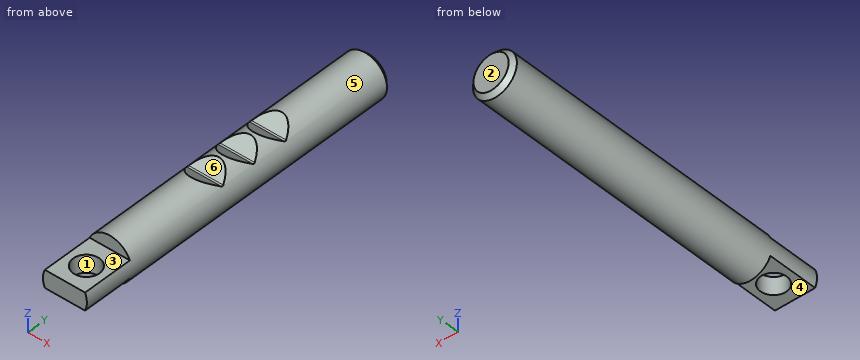
```python
from build123d import *

# Parameters (mm, degrees)
F0_R          = 10
F1_DEPTH      = 156
F2_SIZE       = 2
F3_W          = 20
F3_H          = 8
F4_DEPTH      = 23
F5_R          = 6
F6_DEPTH      = 10.001
F6_DEPTH_BACK = 10.001
F8_DEPTH      = 10.001
F8_DEPTH_BACK = 10.001


# Not quite as in the source:
# - a pattern or mirror of a feature is missing from the dataset's text; its kind, count and spacing are read off the source's solid


with BuildPart() as f1:
    # F0 (on Front) → F1 (new body)
    with BuildSketch(Plane.XZ):
        Circle(F0_R)
    extrude(amount=-F1_DEPTH)

    # F2
    f2_edges = [f1.edges().sort_by_distance(p)[0] for p in [
        (-10, 156, 0),
    ]]
    chamfer(f2_edges, length=F2_SIZE)

    # F3 (on Front) → F4 (cut)
    with BuildSketch(Plane.XZ):
        with Locations((0, 8)):
            Rectangle(F3_W, F3_H)
    f4 = extrude(amount=-F4_DEPTH, mode=Mode.SUBTRACT)

    # F4_copies: F4 across plane
    add(f4.mirror(Plane(origin=(0, 0, 0), x_dir=(-1, 0, 0), z_dir=(0, 0, -1))), mode=Mode.SUBTRACT)

    # F5 (on Top) → F6 (cut, two sides)
    with BuildSketch(Plane.XY) as f6_sk:
        with Locations((0, 11)):
            Circle(F5_R)
    extrude(amount=-F6_DEPTH, mode=Mode.SUBTRACT)
    extrude(f6_sk.sketch, amount=F6_DEPTH_BACK, mode=Mode.SUBTRACT)

    # F7 (on Right) → F8 (cut, two sides)
    with BuildSketch(Plane.YZ) as f8_sk:
        with BuildLine():
            Line((96.0621778265, 10.5), (79.9378221735, 10.5))
            Line((79.9378221735, 10.5), (87.5, 6.1339745962))
            ThreePointArc((87.5, 6.1339745962), (88, 6), (88.5, 6.1339745962))
            Line((88.5, 6.1339745962), (96.0621778265, 10.5))
        make_face()
        with BuildLine():
            Line((112.1865334795, 10.5), (96.0621778265, 10.5))
            Line((96.0621778265, 10.5), (103.624355653, 6.1339745962))
            ThreePointArc((103.624355653, 6.1339745962), (104.124355653, 6), (104.624355653, 6.1339745962))
            Line((104.624355653, 6.1339745962), (112.1865334795, 10.5))
        make_face()
        with BuildLine():
            Line((72.375644347, 6.1339745962), (79.9378221735, 10.5))
            Line((79.9378221735, 10.5), (63.8134665205, 10.5))
            Line((63.8134665205, 10.5), (71.375644347, 6.1339745962))
            ThreePointArc((71.375644347, 6.1339745962), (71.875644347, 6), (72.375644347, 6.1339745962))
        make_face()
    extrude(amount=-F8_DEPTH, mode=Mode.SUBTRACT)
    extrude(f8_sk.sketch, amount=F8_DEPTH_BACK, mode=Mode.SUBTRACT)


solid = f1.part
```
The listing builds one solid part. Answer for the finished solid, in the listing's coordinates (mm). Face numbers are marked on the shaded views. A direction names the side the tool comes from. Round coordinates to 2 decimals unless told otherwise and drop trailing zeros. Loops run counter-clockwise (first coordinate to the right, second up) from the corner with the lowest first, then second, coordinate; pieces in that order, holes last. Notation, with made-up numbers: (27.5, 32.5) - (38.5, 32.5) arc R28 ccw to (38.5, 68.5) - close; hole circle Ø7 at (68.5, 6). An arc over 180 degrees is marked (long way). Return JSON: item names as keys, results as strings. Group by question number.
1. The part is cut by section D-D on y = 131.5. Determine the outline of the cut face in (x, z), then the cut area to 3 significant figures.
2. Each of these flat-tipped pins is pushed along its axis until it touches: P1, Ø12, axis at x = -3.5, z = 1.5, coming from the -Y side; P2, Ø1.5, axis at x = 4.5, z = 5.5, coming from the -Y side; P3, Ø1.5, axis at y = 138.5, z = 4, coming from the -X side; P4, Ø10, axis at x = -7.5, y = 84.5, coming from the +Z side. Where does it stop, or does it pass through?
3. The part is cut by section C-C on z = 0. Determine the outline of the cut face in (x, y), then the cut area to 3 significant figures.
4. Consider probe 1 along X at (y, z) = (11, 0.5); probe 2 along Y at (x, z) = (0, 1.5); probe 3 along Y at (x, z) = (-4, 7.75). Determine where each line is inside the solid, lowest interval first.
5. The part is cut by section B-B on x = 0. Determine the outline of the cut face in (y, z), then the cut area to 3 significant figures.
6. The mould has two halves that part along Y. Classify the marked faces 1, 2 and 3: pulls with the +Y half, pulls with the -Y half, needs draft (parallel to the pull), parting line crosses it, or undercut.
7. The part is cut by section A-A on y = 11. Determine the outline of the cut face in (x, z).
8. Which of the six approach directions +Z, -Z, +X, -X, +Y, -Y give full straight-line access (tool end or side, diameter ignored) to the marked faces 4, 5 and 6?
Resolved:
{
 "1": {"outline": "circle Ø20 at (0, 0)", "area": "314 mm²"},
 "2": {"P1": "stops at y = 0", "P2": "stops at y = 23", "P3": "stops at x = -9.46", "P4": "stops at z = 9.44"},
 "3": {"outline": "(-10, 0) - (10, 0) - (10, 154) - (8, 156) - (-8, 156) - (-10, 154) - close; hole circle Ø12 at (0, 11)", "area": "3,000 mm²"},
 "4": {"probe 1": "x = -9.99 to -6, 6 to 9.99", "probe 2": "y = 0 to 5, 17 to 156", "probe 3": "y = 23 to 68.58, 75.17 to 84.7, 91.3 to 100.83, 107.42 to 155.28"},
 "5": {"outline": "(0, -4) - (5, -4) - (5, 4) - (0, 4) - close; (17, -4) - (23, -4) - (23, -10) - (154, -10) - (156, -8) - (156, 8) - (154, 10) - (111.32, 10) - (104.62, 6.13) arc R1 cw to (103.62, 6.13) - (96.93, 10) - (95.2, 10) - (88.5, 6.13) arc R1 cw to (87.5, 6.13) - (80.8, 10) - (79.07, 10) - (72.38, 6.13) arc R1 cw to (71.38, 6.13) - (64.68, 10) - (23, 10) - (23, 4) - (17, 4) - close", "area": "2,650 mm²"},
 "6": {"face 1": "undercut", "face 2": "pulls with the +Y half", "face 3": "needs draft"},
 "7": {"outline": "(-9.17, -4) - (-6, -4) - (-6, 4) - (-9.17, 4) arc R10 ccw to start; (6, -4) - (9.17, -4) arc R10 ccw to (9.17, 4) - (6, 4) - close"},
 "8": {"face 4": "-Z, +X, -X, -Y", "face 5": "+Y, -Y", "face 6": "+Z, +X, -X"}
}
